from build123d import *

# Parameters (mm, degrees)
SKETCH1_R           = 80
SKETCH1_R_2         = 2.5
BOSS_EXTRUDE1_DEPTH = 4
CUT_EXTRUDE1_DEPTH  = 114.207773585
SKETCH3_R           = 5
CUT_EXTRUDE2_DEPTH  = 3
BOSS_EXTRUDE2_START = 1
SKETCH4_R           = 80
SKETCH4_R_2         = 2.5
SKETCH4_R_3         = 5
BOSS_EXTRUDE2_DEPTH = 1
SKETCH5_R           = 10.6
CUT_EXTRUDE3_DEPTH  = 2.5


with BuildPart() as part:
    # Sketch1 → Boss-Extrude1 (new body)
    with BuildSketch(Plane(origin=(0, 0, 0), x_dir=(1, 0, 0), z_dir=(0, 1, 0))):
        with Locations(Location((0, 0, 0), (0, 0, 270))):
            Circle(SKETCH1_R)
        with Locations(Location((-15, 15, 0), (0, 0, 270))):
            Circle(SKETCH1_R_2, mode=Mode.SUBTRACT)
        with Locations(Location((15, 15, 0), (0, 0, 270))):
            Circle(SKETCH1_R_2, mode=Mode.SUBTRACT)
        with Locations(Location((15, -15, 0), (0, 0, 270))):
            Circle(SKETCH1_R_2, mode=Mode.SUBTRACT)
        with Locations(Location((-15, -15, 0), (0, 0, 270))):
            Circle(SKETCH1_R_2, mode=Mode.SUBTRACT)
    extrude(amount=BOSS_EXTRUDE1_DEPTH)

    # Sketch2 → Cut-Extrude1 (cut, through all)
    with BuildSketch(Plane(origin=(0, 4, 0), x_dir=(1, 0, 0), z_dir=(0, 1, 0))):
        Polygon((4, 72.309401077), (4, 67.690598923), (0, 65.381197846), (-4, 67.690598923), (-4, 72.309401077), (0, 74.618802154), align=None)
        Polygon((45.738467533, 56.148393315), (43.023603743, 52.411703879), (38.430103871, 52.89450017), (36.551467788, 57.113985897), (39.266331578, 60.850675333), (43.85983145, 60.367879042), align=None)
        Polygon((70.006395061, 18.540607721), (65.613653175, 17.113319362), (62.181214255, 20.203901247), (63.14151722, 24.721771492), (67.534259106, 26.149059851), (70.966698026, 23.058477965), align=None)
        Polygon((67.534259106, -26.149059851), (63.14151722, -24.721771492), (62.181214255, -20.203901247), (65.613653175, -17.113319362), (70.006395061, -18.540607721), (70.966698026, -23.058477965), align=None)
        Polygon((39.266331578, -60.850675333), (36.551467788, -57.113985897), (38.430103871, -52.89450017), (43.023603743, -52.411703879), (45.738467533, -56.148393315), (43.85983145, -60.367879042), align=None)
        Polygon((-4, -72.309401077), (-4, -67.690598923), (0, -65.381197846), (4, -67.690598923), (4, -72.309401077), (0, -74.618802154), align=None)
        Polygon((-45.738467533, -56.148393315), (-43.023603743, -52.411703879), (-38.430103871, -52.89450017), (-36.551467788, -57.113985897), (-39.266331578, -60.850675333), (-43.85983145, -60.367879042), align=None)
        Polygon((-70.006395061, -18.540607721), (-65.613653175, -17.113319362), (-62.181214255, -20.203901247), (-63.14151722, -24.721771492), (-67.534259106, -26.149059851), (-70.966698026, -23.058477965), align=None)
        Polygon((-67.534259106, 26.149059851), (-63.14151722, 24.721771492), (-62.181214255, 20.203901247), (-65.613653175, 17.113319362), (-70.006395061, 18.540607721), (-70.966698026, 23.058477965), align=None)
        Polygon((-39.266331578, 60.850675333), (-36.551467788, 57.113985897), (-38.430103871, 52.89450017), (-43.023603743, 52.411703879), (-45.738467533, 56.148393315), (-43.85983145, 60.367879042), align=None)
    extrude(amount=-CUT_EXTRUDE1_DEPTH, mode=Mode.SUBTRACT)

    # Sketch3 → Cut-Extrude2 (cut)
    with BuildSketch(Plane(origin=(0, 4, 0), x_dir=(1, 0, 0), z_dir=(0, 1, 0))):
        with Locations(Location((-15, -15, 0), (0, 0, 270))):
            Circle(SKETCH3_R)
        with Locations(Location((15, -15, 0), (0, 0, 270))):
            Circle(SKETCH3_R)
        with Locations(Location((15, 15, 0), (0, 0, 270))):
            Circle(SKETCH3_R)
        with Locations(Location((-15, 15, 0), (0, 0, 270))):
            Circle(SKETCH3_R)
    extrude(amount=-CUT_EXTRUDE2_DEPTH, mode=Mode.SUBTRACT)

    # Sketch4 → Boss-Extrude2 (add)
    with BuildSketch(Plane(origin=(0, 4, 0), x_dir=(1, 0, 0), z_dir=(0, 1, 0)).offset(BOSS_EXTRUDE2_START)):
        with Locations(Location((0, 0, 0), (0, 0, 270))):
            Circle(SKETCH4_R)
        with Locations(Location((41.14496766, 56.631189606, 0), (0, 0, 270))):
            Circle(SKETCH4_R_2, mode=Mode.SUBTRACT)
        with Locations(Location((0, 70, 0), (0, 0, 270))):
            Circle(SKETCH4_R_2, mode=Mode.SUBTRACT)
        with Locations(Location((66.573956141, 21.631189606, 0), (0, 0, 270))):
            Circle(SKETCH4_R_2, mode=Mode.SUBTRACT)
        with Locations(Location((66.573956141, -21.631189606, 0), (0, 0, 270))):
            Circle(SKETCH4_R_2, mode=Mode.SUBTRACT)
        with Locations(Location((-15, 15, 0), (0, 0, 270))):
            Circle(SKETCH4_R_3, mode=Mode.SUBTRACT)
        with Locations(Location((41.14496766, -56.631189606, 0), (0, 0, 270))):
            Circle(SKETCH4_R_2, mode=Mode.SUBTRACT)
        with Locations(Location((15, 15, 0), (0, 0, 270))):
            Circle(SKETCH4_R_3, mode=Mode.SUBTRACT)
        with Locations(Location((0, -70, 0), (0, 0, 270))):
            Circle(SKETCH4_R_2, mode=Mode.SUBTRACT)
        with Locations(Location((-15, -15, 0), (0, 0, 270))):
            Circle(SKETCH4_R_3, mode=Mode.SUBTRACT)
        with Locations(Location((-41.14496766, -56.631189606, 0), (0, 0, 270))):
            Circle(SKETCH4_R_2, mode=Mode.SUBTRACT)
        with Locations(Location((15, -15, 0), (0, 0, 270))):
            Circle(SKETCH4_R_3, mode=Mode.SUBTRACT)
        with Locations(Location((-66.573956141, -21.631189606, 0), (0, 0, 270))):
            Circle(SKETCH4_R_2, mode=Mode.SUBTRACT)
        with Locations(Location((-66.573956141, 21.631189606, 0), (0, 0, 270))):
            Circle(SKETCH4_R_2, mode=Mode.SUBTRACT)
        with Locations(Location((-41.14496766, 56.631189606, 0), (0, 0, 270))):
            Circle(SKETCH4_R_2, mode=Mode.SUBTRACT)
    extrude(amount=-BOSS_EXTRUDE2_DEPTH)

    # Sketch5 → Cut-Extrude3 (cut)
    with BuildSketch(Plane(origin=(0, 5, 0), x_dir=(1, 0, 0), z_dir=(0, 1, 0))):
        with Locations(Location((0, 0, 0), (0, 0, 270))):
            Circle(SKETCH5_R)
    extrude(amount=-CUT_EXTRUDE3_DEPTH, mode=Mode.SUBTRACT)


solid = part.part
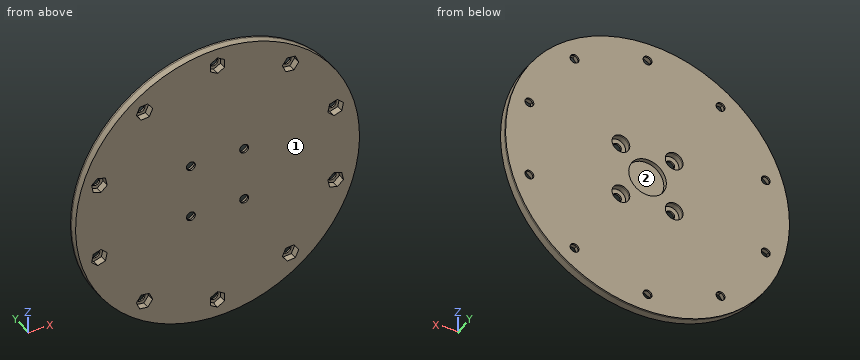
Can you work these out from the model? Positions are in its coordinate system, mm. Face numbers are marked on the shaded views. Give positions to 0.01 mm unless a question says otherwise; leave off trailing zeros. Loops run counter-clockwise (first coordinate to the right, second up) from the corner with the lowest first, then second, coordinate; pieces in that order, holes last. Notation, with made-up numbers: (12.25, 19) - (50.25, 19) arc R23 cw to (50.25, 57) - close; hole circle Ø9 at (-14, 68). An arc over 180 degrees is marked (long way). One line per item, written item: value.
(1) If we mould it in two halves opening along X, with no side actions, what happens to the marked faces 1 and 2? For each: released by +X, released by -X, zero draft, split by the parting line, or undercut.
Verdict:
face 1: zero draft
face 2: undercut
(2) If we section it at B-B, the plane x = -15: List the corners of the cut face in (y, z) for me.
Verdict:
outline: (0, -78.58) - (5, -78.58) - (5, -20) - (1, -20) - (1, -17.5) - (0, -17.5) - close; (0, -12.5) - (1, -12.5) - (1, -10) - (5, -10) - (5, 10) - (1, 10) - (1, 12.5) - (0, 12.5) - close; (0, 17.5) - (1, 17.5) - (1, 20) - (5, 20) - (5, 78.58) - (0, 78.58) - close
(3) If we section it at A-A, the plane z = -70: List the corners of the cut face in (x, y) for me.
Verdict:
outline: (-38.73, 0) - (-4, 0) - (-4, 4) - (-2.5, 4) - (-2.5, 5) - (-38.73, 5) - close; (2.5, 4) - (4, 4) - (4, 0) - (38.73, 0) - (38.73, 5) - (2.5, 5) - close
(4) I need wall thicknesses on line 1 along X through (y, z) = (4.55, -15); line 2 along X through (y, z) = (4.45, 0); line 3 along Z through (x, y) = (-3, 0.65). Which ranges of each line are inside material? Lowest first, please.
Verdict:
line 1: -78.58 to -20, -10 to 10, 20 to 78.58
line 2: -80 to -10.6, 10.6 to 80
line 3: -79.94 to -72.89, -67.11 to 67.11, 72.89 to 79.94
(5) If we section it at C-C, the plane z = -15: List the corners of the cut face in (x, y) for me, plus the area to 3 significant figures.
Verdict:
outline: (-78.58, 0) - (-17.5, 0) - (-17.5, 1) - (-20, 1) - (-20, 5) - (-78.58, 5) - close; (-12.5, 0) - (12.5, 0) - (12.5, 1) - (10, 1) - (10, 5) - (-10, 5) - (-10, 1) - (-12.5, 1) - close; (17.5, 0) - (78.58, 0) - (78.58, 5) - (20, 5) - (20, 1) - (17.5, 1) - close
area: 696 mm^2
(6) I'm going to push flat-ended pins straight in: pin 1 (17 mm diameter, centred on x = 4, z = -1.5, fed in from +Y); pin 2 (6 mm diameter, centred on x = -15, z = -15, fed in from +Y); pin 3 (4 mm diameter, centred on x = 66.57, z = 21.63, fed in from -Y); pin 4 (1.2 mm diameter, centred on y = 2, z = 70, fed in from +X) (3 decimals). Where does each tip first touch, or does it pass through?
Verdict:
pin 1: y = 5
pin 2: y = 1
pin 3: through
pin 4: x = 39.795
(7) If we section it at D-D, the plane x = -32.5: List the corners of the cut face in (y, z) for me.
Verdict:
outline: (0, -73.1) - (5, -73.1) - (5, 73.1) - (0, 73.1) - close
